Verification items for the finished model (mm, model axes). A direction names the side the tool comes from. Round coordinates to 2 decimals unless told otherwise and drop trailing zeros. Write each loop counter-clockwise with the first axis right and the second up, starting at its lowest first coordinate (ties: lowest second). Pieces come first, ordered by that corner, then holes. Notation, with made-up numbers: (-27, 59) - (31, 59) arc R23 cw to (31, 88) - close; hole circle Ø10 at (0.5, 46.5). An arc over 180 degrees is marked (long way). Answer as a JSON object with one key per item and string values.
```python
from build123d import *

# Parameters (mm, degrees)
ESBO_O1_W                = 50
ESBO_O1_H                = 35
ESBO_O1_R                = 5.25
ESBO_O1_R_2              = 1.75
RESSALTO_EXTRUS_O1_DEPTH = 6
ESBO_O2_W                = 16
ESBO_O2_H                = 6
ESBO_O2_W_2              = 5
CORTE_EXTRUS_O1_DEPTH    = 6


with BuildPart() as part:
    # Esboço1 → Ressalto-extrusão1 (new body)
    with BuildSketch(Plane.XY):
        Rectangle(ESBO_O1_W, ESBO_O1_H)
        with Locations((0, -2.35)):
            Circle(ESBO_O1_R, mode=Mode.SUBTRACT)
        with Locations((5.656854249, 3.306854249)):
            Circle(ESBO_O1_R_2, mode=Mode.SUBTRACT)
        with Locations((-5.656854249, 3.306854249)):
            Circle(ESBO_O1_R_2, mode=Mode.SUBTRACT)
        with Locations((-5.656854249, -8.006854249)):
            Circle(ESBO_O1_R_2, mode=Mode.SUBTRACT)
        with Locations((5.656854249, -8.006854249)):
            Circle(ESBO_O1_R_2, mode=Mode.SUBTRACT)
    extrude(amount=RESSALTO_EXTRUS_O1_DEPTH)

    # Esboço2 → Corte-extrusão1 (cut)
    with BuildSketch(Plane.XY.offset(6)):
        with Locations((0, 14.5)):
            Rectangle(ESBO_O2_W, ESBO_O2_H)
        with Locations((-22.5, 14.5)):
            Rectangle(ESBO_O2_W_2, ESBO_O2_H)
        with Locations((22.5, 14.5)):
            Rectangle(ESBO_O2_W_2, ESBO_O2_H)
    extrude(amount=-CORTE_EXTRUS_O1_DEPTH, mode=Mode.SUBTRACT)


solid = part.part
```
1. Access from +Z, -Z, +X, -X, +Y, -Y to the whole of each face (thin tool, end or side, straight path). Record for faces 1 (the face through (-8, 14, 3)), 2 (the face through (7.326, 3.833, 2.958)), 3 (the face through (-20, 14, 3)), 4 (the face through (14, 17.5, 3)), 5 (the face through (22, 11.5, 3)).
Completed:
{"face 1": "+Z, -Z, +Y", "face 2": "+Z, -Z", "face 3": "+Z, -Z, -X, +Y", "face 4": "+Z, -Z, +X, -X, +Y", "face 5": "+Z, -Z, +X, +Y"}
2. Cross-section at A-A (x = 0). Record the boundary of the cut face in (y, z).
Completed:
{"outline": "(-17.5, 0) - (-7.6, 0) - (-7.6, 6) - (-17.5, 6) - close; (2.9, 0) - (11.5, 0) - (11.5, 6) - (2.9, 6) - close"}
3. Go/stop test with flat-tipped pins: pin 1 (3 mm diameter, centred on x = -5.66, y = -8.01, fed in from +Z); pin 2 (1.8 mm diameter, centred on x = 1, z = 1.5, fed in from +Y); pin 3 (1.5 mm diameter, centred on x = 2, y = 4.5, fed in from -Z); pin 4 (1.8 mm diameter, centred on y = 14, z = 3.5, fed in from +X). Record where each tip stops, or that it passes through.
Completed:
{"pin 1": "passes through", "pin 2": "stops at y = 11.5", "pin 3": "stops at z = 0", "pin 4": "stops at x = 20"}
4. Material ranges on probe 1 along X at (y, z) = (15, 1.7); probe 2 along X at (y, z) = (-9, 5.55); probe 3 along X at (y, z) = (-8, 1.3), recorded low to high. Write a range as from..to.
Completed:
{"probe 1": "x = -20..-8, 8..20", "probe 2": "x = -25..-7.1, -4.22..4.22, 7.1..25", "probe 3": "x = -25..-7.41, -3.91..3.91, 7.41..25"}
5. Cross-section at C-C (z = 5.2). Record the boundary of the cut face in (x, y), plus the area to 3 significant figures.
Completed:
{"outline": "(-25, -17.5) - (25, -17.5) - (25, 11.5) - (20, 11.5) - (20, 17.5) - (8, 17.5) - (8, 11.5) - (-8, 11.5) - (-8, 17.5) - (-20, 17.5) - (-20, 11.5) - (-25, 11.5) - close; hole circle Ø3.5 at (-5.66, -8.01); hole circle Ø3.5 at (-5.66, 3.31); hole circle Ø10.5 at (0, -2.35); hole circle Ø3.5 at (5.66, -8.01); hole circle Ø3.5 at (5.66, 3.31)", "area": "1,470 mm^2"}
6. Mould release check, pull along X, two halves, no side actions. Record for faces 6 (the face through (-14, 17.5, 3)), 7 (the face through (0, 11.5, 3)), 8 (the face through (25, -3, 3)): released by +X, released by -X, zero draft, split by the parting line, or undercut.
Completed:
{"face 6": "zero draft", "face 7": "undercut", "face 8": "released by +X"}
7. Cross-section at B-B (y = 15). Record the boundary of the cut face in (x, z).
Completed:
{"outline": "(-20, 0) - (-8, 0) - (-8, 6) - (-20, 6) - close; (8, 0) - (20, 0) - (20, 6) - (8, 6) - close"}
